```python
from build123d import *

# Parameters (mm, degrees)
EXTRUDE_1_DEPTH     = 1.63
SKETCH_2_R          = 1.5
CUT_EXTRUDE_1_DEPTH = 1.6
SKETCH_3_W          = 34.52
SKETCH_3_H          = 23.21
EXTRUDE_2_DEPTH     = 1.8
EXTRUDE_3_DEPTH     = 2
SKETCH_4_W          = 5.81
SKETCH_4_H          = 3.67
EXTRUDE_4_DEPTH     = 2
SKETCH_7_W          = 2.6
SKETCH_7_H          = 1.3
EXTRUDE_5_DEPTH     = 1
SKETCH_8_W          = 51
SKETCH_8_H          = 5
EXTRUDE_6_DEPTH     = 3.68
SKETCH_9_W          = 1.9
SKETCH_9_H          = 1.9
EXTRUDE_7_DEPTH     = 3
SKETCH_10_R         = 1.6
EXTRUDE_8_DEPTH     = 1
SKETCH_11_W         = 34.52
SKETCH_11_H         = 5
CUT_EXTRUDE_2_DEPTH = 0.2


with BuildPart() as part:
    # 草图1 → 凸台-拉伸1 (new body)
    with BuildSketch(Plane(origin=(0, 0, 0), x_dir=(1, 0, 0), z_dir=(0, 1, 0))):
        with BuildLine():
            Line((-29.5, 15.375), (29.5, 15.375))
            ThreePointArc((29.5, 15.375), (31.621320344, 14.496320344), (32.5, 12.375))
            Line((32.5, 12.375), (32.5, -12.375))
            ThreePointArc((32.5, -12.375), (31.621320344, -14.496320344), (29.5, -15.375))
            Line((29.5, -15.375), (-29.5, -15.375))
            ThreePointArc((-29.5, -15.375), (-31.621320344, -14.496320344), (-32.5, -12.375))
            Line((-32.5, -12.375), (-32.5, 12.375))
            ThreePointArc((-32.5, 12.375), (-31.621320344, 14.496320344), (-29.5, 15.375))
        make_face()
    extrude(amount=EXTRUDE_1_DEPTH)

    # 草图2 → 切除-拉伸1 (cut)
    with BuildSketch(Plane(origin=(0, 1.63, 0), x_dir=(1, 0, 0), z_dir=(0, 1, 0))):
        with Locations(Location((-29, 11.875, 0), (0, 0, 270))):  # turned: the seam where the file's is
            Circle(SKETCH_2_R)
        with Locations(Location((-29, -11.875, 0), (0, 0, 270))):  # turned: the seam where the file's is
            Circle(SKETCH_2_R)
        with Locations(Location((29, -11.875, 0), (0, 0, 270))):  # turned: the seam where the file's is
            Circle(SKETCH_2_R)
        with Locations(Location((29, 11.875, 0), (0, 0, 270))):  # turned: the seam where the file's is
            Circle(SKETCH_2_R)
    extrude(amount=-CUT_EXTRUDE_1_DEPTH, mode=Mode.SUBTRACT)

    # 草图3 → 凸台-拉伸2 (add)
    with BuildSketch(Plane(origin=(0, 1.63, 0), x_dir=(1, 0, 0), z_dir=(0, 1, 0))):
        with Locations((0.48, -1.24)):
            Rectangle(SKETCH_3_W, SKETCH_3_H)
    extrude(amount=EXTRUDE_2_DEPTH)

    # 草图5 → 凸台-拉伸3 (add)
    with BuildSketch(Plane(origin=(0, 1.63, 0), x_dir=(1, 0, 0), z_dir=(0, 1, 0))):
        with BuildLine():
            Line((26.024695167, 3.538250353), (28.464213562, 1.098731957))
            ThreePointArc((28.464213562, 1.098731957), (29.05, -0.315481605), (28.464213562, -1.729695167))
            Line((28.464213562, -1.729695167), (26.024695167, -4.169213562))
            ThreePointArc((26.024695167, -4.169213562), (24.610481605, -4.755), (23.196268043, -4.169213562))
            Line((23.196268043, -4.169213562), (20.756749647, -1.729695167))
            ThreePointArc((20.756749647, -1.729695167), (20.17096321, -0.315481605), (20.756749647, 1.098731957))
            Line((20.756749647, 1.098731957), (23.196268043, 3.538250353))
            ThreePointArc((23.196268043, 3.538250353), (24.610481605, 4.12403679), (26.024695167, 3.538250353))
        make_face()
    extrude(amount=EXTRUDE_3_DEPTH)

    # 草图4 → 凸台-拉伸4 (add)
    with BuildSketch(Plane(origin=(0, 1.63, 0), x_dir=(1, 0, 0), z_dir=(0, 1, 0))):
        with Locations((-24.325, 6.45)):
            Rectangle(SKETCH_4_W, SKETCH_4_H)
        with Locations((-24.325, 0.18)):
            Rectangle(SKETCH_4_W, SKETCH_4_H)
        with Locations((-24.325, -6.09)):
            Rectangle(SKETCH_4_W, SKETCH_4_H)
    extrude(amount=EXTRUDE_4_DEPTH)

    # 草图7 → 凸台-拉伸5 (add)
    with BuildSketch(Plane(origin=(0, 3.63, 0), x_dir=(1, 0, 0), z_dir=(0, 1, 0))):
        with Locations((-24.325, 6.45)):
            Rectangle(SKETCH_7_W, SKETCH_7_H)
        with Locations((-24.325, 0.18)):
            Rectangle(SKETCH_7_W, SKETCH_7_H)
        with Locations((-24.325, -6.09)):
            Rectangle(SKETCH_7_W, SKETCH_7_H)
    extrude(amount=EXTRUDE_5_DEPTH)

    # 草图8 → 凸台-拉伸6 (add)
    with BuildSketch(Plane.XZ):
        with Locations((-0.2, -11.235)):
            Rectangle(SKETCH_8_W, SKETCH_8_H)
    extrude(amount=EXTRUDE_6_DEPTH)

    # 草图9 → 凸台-拉伸7 (add)
    with BuildSketch(Plane(origin=(0, 3.63, 0), x_dir=(1, 0, 0), z_dir=(0, 1, 0))):
        with Locations((24.610481605, -0.315481605)):
            Rectangle(SKETCH_9_W, SKETCH_9_H)
    extrude(amount=EXTRUDE_7_DEPTH)

    # 草图10 → 凸台-拉伸8 (add)
    with BuildSketch(Plane(origin=(0, 3.63, 0), x_dir=(1, 0, 0), z_dir=(0, 1, 0))):
        with Locations(Location((24.610481605, -0.315481605, 0), (0, 0, 90))):  # turned: the seam where the file's is
            Circle(SKETCH_10_R)
    extrude(amount=EXTRUDE_8_DEPTH)

    # 草图11 → 切除-拉伸2 (cut)
    with BuildSketch(Plane(origin=(0, 3.43, 0), x_dir=(1, 0, 0), z_dir=(0, 1, 0))):
        with Locations((0.48, -10.345)):
            Rectangle(SKETCH_11_W, SKETCH_11_H)
    extrude(amount=-CUT_EXTRUDE_2_DEPTH, mode=Mode.SUBTRACT)


solid = part.part
```
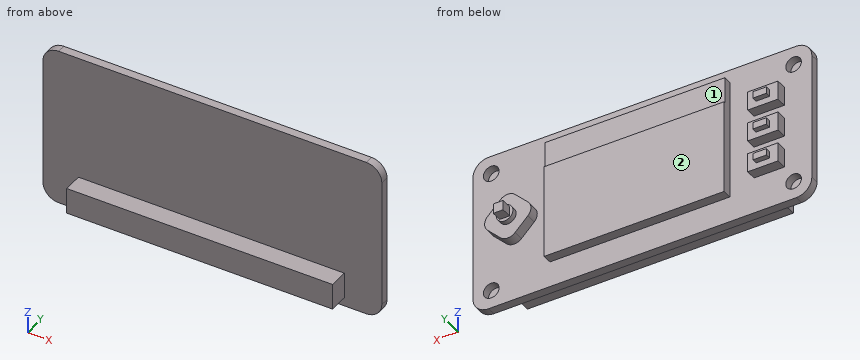
Verification items for the finished model (mm, model axes). Face numbers are marked on the shaded views. Round coordinates to 2 decimals unless told otherwise and drop trailing zeros. Write each loop counter-clockwise with the first axis right and the second up, starting at its lowest first coordinate (ties: lowest second). Pieces come first, ordered by that corner, then holes. Notation, with made-up numbers: (-20, -27) - (10, -27) arc R35 cw to (10, 7) - close; hole circle Ø5 at (-24.5, 12). An arc over 180 degrees is marked (long way). Answer as a JSON object with one key per item and string values. Group by question number.
Q1. Section check A-A, the plane x = -26.5. Enter the section's corners in (y, z) (3 decimals), plus the area to 3 significant figures.
Q2. Go/stop test with flat-tipped pins: pin 1 Ø8 at (x, z) = (11, 10) entering from +Y; pin 2 Ø1.1 at (x, z) = (-25, -7) entering from +Y; pin 3 Ø1.1 at (x, y) = (-6, -1.5) entering from +Z (3 decimals); pin 4 Ø3 at (y, z) = (-2, -3.5) entering from -X. Record where each tip stops, or that it passes through.
Q3. Mould release check, pull along X, two halves, no side actions. Record for the marked faces 1 and 2: released by +X, released by -X, zero draft, split by the parting line, or undercut.
Q4. Section check B-B, the plane z = 3. Enter the section's corners in (x, y).
Q5. Section check C-C, the plane y = -1.5. Enter the section's corners in (x, z) (3 decimals), plus the area to 3 significant figures.
Q6. Section check D-D, the plane z = 11. Enter the section's corners in (x, y).
Q7. Thickness scan on line 1 (Y direction, x = -21.5, z = 8.5); line 2 (X direction, y = -1.5, z = -10.5); line 3 (X direction, y = 3, z = 12). Record the ranges inside material, lowest first.
Found:
{
 "1": {"outline": "(0, -15.375) - (1.63, -15.375) - (1.63, -8.285) - (3.63, -8.285) - (3.63, -4.615) - (1.63, -4.615) - (1.63, -2.015) - (3.63, -2.015) - (3.63, 1.655) - (1.63, 1.655) - (1.63, 4.255) - (3.63, 4.255) - (3.63, 7.925) - (1.63, 7.925) - (1.63, 15.375) - (0, 15.375) - close", "area": "72.1 mm^2"},
 "2": {"pin 1": "stops at y = 3.43", "pin 2": "stops at y = 4.63", "pin 3": "stops at z = -8.735", "pin 4": "passes through"},
 "3": {"face 1": "zero draft", "face 2": "undercut"},
 "4": {"outline": "(-32.5, 0) - (32.5, 0) - (32.5, 1.63) - (27.19, 1.63) - (27.19, 3.63) - (22.03, 3.63) - (22.03, 1.63) - (17.74, 1.63) - (17.74, 3.43) - (-16.78, 3.43) - (-16.78, 1.63) - (-32.5, 1.63) - close"},
 "5": {"outline": "(-25.7, -13.735) - (25.3, -13.735) - (25.3, -8.735) - (-25.7, -8.735) - close", "area": "255 mm^2"},
 "6": {"outline": "(-32.5, 0) - (32.5, 0) - (32.5, 1.63) - (30.22, 1.63) - (30.22, 0.03) - (27.78, 0.03) - (27.78, 1.63) - (17.74, 1.63) - (17.74, 3.23) - (-16.78, 3.23) - (-16.78, 1.63) - (-27.78, 1.63) - (-27.78, 0.03) - (-30.22, 0.03) - (-30.22, 1.63) - (-32.5, 1.63) - close"},
 "7": {"line 1": "y = 0 to 1.63", "line 2": "x = -25.7 to 25.3", "line 3": "x = -16.78 to 17.74"}
}
